```python
from build123d import *

# Parameters (mm, degrees)
SKETCH1_W            = 6
SKETCH1_H            = 6
EXTRUDE1_DEPTH       = 3.4
SKETCH2_W            = 1.5
SKETCH2_H            = 3
SKETCH2_H_2          = 0.5
SKETCH2_W_2          = 2
SKETCH2_H_3          = 6
SKETCH2_W_3          = 1
EXTRUDE2_DEPTH       = 0.4
REVOLVE1_ANGLE       = 180
LPATTERN1_COUNT      = 2
LPATTERN1_PITCH      = 4.5
LPATTERN1_COUNT_DIR2 = 2
LPATTERN1_PITCH_DIR2 = 4.5
SKETCH4_R            = 1.8
EXTRUDE3_DEPTH       = 6.1
EXTRUDE3_TAPER       = 2
EXTRUDE4_DEPTH       = 0.375
MIRROR2_COPY_1_DEPTH = 0.375
FILLET1_R            = 0.25


with BuildPart() as part:
    # Sketch1 → Extrude1 (new body)
    with BuildSketch(Plane(origin=(0, 0, 0), x_dir=(1, 0, 0), z_dir=(0, 1, 0))):
        Rectangle(SKETCH1_W, SKETCH1_H)
    extrude(amount=EXTRUDE1_DEPTH)

    # Sketch2 → Extrude2 (cut)
    with BuildSketch(Plane.XZ):
        with Locations((-2.25, 0)):
            Rectangle(SKETCH2_W, SKETCH2_H)
        with Locations((-2.25, -2.75)):
            Rectangle(SKETCH2_W, SKETCH2_H_2)
        with Locations((-2.25, 2.75)):
            Rectangle(SKETCH2_W, SKETCH2_H_2)
        Rectangle(SKETCH2_W_2, SKETCH2_H_3)
        with Locations((0, -2.25)):
            Rectangle(SKETCH2_W_3, SKETCH2_H_2, mode=Mode.SUBTRACT)
        with Locations((0, 2.25)):
            Rectangle(SKETCH2_W_3, SKETCH2_H_2, mode=Mode.SUBTRACT)
        Rectangle(SKETCH2_W_3, SKETCH2_H_2, mode=Mode.SUBTRACT)
        with Locations((2.25, 2.75)):
            Rectangle(SKETCH2_W, SKETCH2_H_2)
        with Locations((2.25, -2.75)):
            Rectangle(SKETCH2_W, SKETCH2_H_2)
        with Locations((2.25, 0)):
            Rectangle(SKETCH2_W, SKETCH2_H)
    extrude(amount=-EXTRUDE2_DEPTH, mode=Mode.SUBTRACT)

    # Sketch3 → Revolve1 (revolve)
    with BuildSketch(Plane(origin=(0, 3.4, 0), x_dir=(1, 0, 0), z_dir=(0, 1, 0))):
        with BuildLine():
            Line((-2.25, 1.75), (-2.25, 2.75))
            ThreePointArc((-2.25, 2.75), (-2.75, 2.25), (-2.25, 1.75))
        make_face()
    revolve1 = revolve(axis=Axis((-2.25, 3.4, -1.75), (0, 0, -1)), revolution_arc=REVOLVE1_ANGLE)

    # LPattern1: Revolve1 2 × 2
    with Locations(*[(i * LPATTERN1_PITCH, 0, j * LPATTERN1_PITCH_DIR2) for i in range(LPATTERN1_COUNT) for j in range(LPATTERN1_COUNT_DIR2) if (i, j) != (0, 0)]):
        add(revolve1)

    # Sketch4 → Extrude3 (add)
    with BuildSketch(Plane(origin=(0, 3.4, 0), x_dir=(1, 0, 0), z_dir=(0, 1, 0))):
        Circle(SKETCH4_R)
    extrude(amount=EXTRUDE3_DEPTH, taper=EXTRUDE3_TAPER)

    # Sketch5 → Extrude4 (add, symmetric)
    with BuildSketch(Plane(origin=(2.25, 0, 0), x_dir=(0, 0, -1), z_dir=(1, 0, 0))):
        with BuildLine():
            Line((3.125, -3.5), (3.125, -3.172113494))
            ThreePointArc((3.125, -3.172113494), (3.171283049, -2.871407695), (3.305847956, -2.598537058))
            Line((3.305847956, -2.598537058), (3.819675491, -1.864715287))
            ThreePointArc((3.819675491, -1.864715287), (3.855845082, -1.75), (3.819675491, -1.635284713))
            Line((3.819675491, -1.635284713), (3.305847956, -0.901462942))
            ThreePointArc((3.305847956, -0.901462942), (3.171283049, -0.628592305), (3.125, -0.327886506))
            Line((3.125, -0.327886506), (3.125, 0.4))
            ThreePointArc((3.125, 0.4), (3.095710678, 0.470710678), (3.025, 0.5))
            Line((3.025, 0.5), (3, 0.5))
            Line((3, 0.5), (3, 0.75))
            Line((3, 0.75), (3.025, 0.75))
            ThreePointArc((3.025, 0.75), (3.272487373, 0.647487373), (3.375, 0.4))
            Line((3.375, 0.4), (3.375, -0.327886506))
            ThreePointArc((3.375, -0.327886506), (3.409712287, -0.553415856), (3.510635967, -0.758068833))
            Line((3.510635967, -0.758068833), (4.024463502, -1.491890604))
            ThreePointArc((4.024463502, -1.491890604), (4.105845082, -1.75), (4.024463502, -2.008109396))
            Line((4.024463502, -2.008109396), (3.510635967, -2.741931167))
            ThreePointArc((3.510635967, -2.741931167), (3.409712287, -2.946584144), (3.375, -3.172113494))
            Line((3.375, -3.172113494), (3.375, -3.5))
            Line((3.375, -3.5), (3.125, -3.5))
        make_face()
    extrude4 = extrude(amount=EXTRUDE4_DEPTH, both=True)

    # Mirror1: Extrude4 across plane
    add(extrude4.mirror(Plane.XY))

    # Mirror2: Extrude4 across plane
    add(extrude4.mirror(Plane(origin=(0, 0, 0), x_dir=(0, 0, 1), z_dir=(1, 0, 0))))

    # Mirror2 copy 1 sketch → Mirror2 copy 1 (add, symmetric)
    with BuildSketch(Plane.ZY.offset(2.25)):
        with BuildLine():
            Line((3.125, -3.5), (3.125, -3.172113494))
            ThreePointArc((3.125, -3.172113494), (3.171283049, -2.871407695), (3.305847956, -2.598537058))
            Line((3.305847956, -2.598537058), (3.819675491, -1.864715287))
            ThreePointArc((3.819675491, -1.864715287), (3.855845082, -1.75), (3.819675491, -1.635284713))
            Line((3.819675491, -1.635284713), (3.305847956, -0.901462942))
            ThreePointArc((3.305847956, -0.901462942), (3.171283049, -0.628592305), (3.125, -0.327886506))
            Line((3.125, -0.327886506), (3.125, 0.4))
            ThreePointArc((3.125, 0.4), (3.095710678, 0.470710678), (3.025, 0.5))
            Line((3.025, 0.5), (3, 0.5))
            Line((3, 0.5), (3, 0.75))
            Line((3, 0.75), (3.025, 0.75))
            ThreePointArc((3.025, 0.75), (3.272487373, 0.647487373), (3.375, 0.4))
            Line((3.375, 0.4), (3.375, -0.327886506))
            ThreePointArc((3.375, -0.327886506), (3.409712287, -0.553415856), (3.510635967, -0.758068833))
            Line((3.510635967, -0.758068833), (4.024463502, -1.491890604))
            ThreePointArc((4.024463502, -1.491890604), (4.105845082, -1.75), (4.024463502, -2.008109396))
            Line((4.024463502, -2.008109396), (3.510635967, -2.741931167))
            ThreePointArc((3.510635967, -2.741931167), (3.409712287, -2.946584144), (3.375, -3.172113494))
            Line((3.375, -3.172113494), (3.375, -3.5))
            Line((3.375, -3.5), (3.125, -3.5))
        make_face()
    extrude(amount=MIRROR2_COPY_1_DEPTH, both=True)

    # Fillet1
    fillet1_edges = [part.edges().sort_by_distance(p)[0] for p in [
        (-1.586983306, 9.5, 0),
        (3, 1.9, 3),
        (-3, 1.9, 3),
        (-3, 1.9, -3),
        (3, 1.9, -3),
        (3, 1.9, 3),
        (-3, 1.9, 3),
        (-3, 1.9, -3),
        (3, 1.9, -3),
    ]]
    fillet(fillet1_edges, radius=FILLET1_R)


solid = part.part
```
Source: CAD feature listing. Evaluate the final solid. Frame: model axes, mm. A direction names the side the tool comes from. Coordinates: 2 decimals unless noted, no trailing zeros. Order: outer loops, then holes, each group sorted by start corner. A loop starts at its lowest first (then second) coordinate and runs counter-clockwise, first axis right, second up. Notation, with made-up numbers: (82, 20.25) - (140, 20.25) arc R14 cw to (140, 29.25) - close; hole circle Ø2 at (12.5, -17). An arc over 180 degrees is marked (long way). One line per item, written item: value.
1) Cut plane B-B on y = 2.5. Output: boundary loops of the cut face in (x, z).
Computed values:
outline: (-3, -2.75) arc R0.25 ccw to (-2.75, -3) - (2.75, -3) arc R0.25 ccw to (3, -2.75) - (3, 2.75) arc R0.25 ccw to (2.75, 3) - (-2.75, 3) arc R0.25 ccw to (-3, 2.75) - close
2) Reachability of faces 1 (the face through (2, 0.4, 0)), 2 (the face through (-1.3, 0, 0)), 3 (the face through (-2, 0.4, 0)), 4 (the face through (0, 9.5, 0)), 5 (the face through (-0.368, 6.37, 1.656)) from +Z, -Z, +X, -X, +Y, -Y: full face, straight path, thin tool, end or side. Return the list, or none.
Computed values:
face 1: +X, -Y
face 2: +X, -X, -Y
face 3: -X, -Y
face 4: +Z, -Z, +X, -X, +Y
face 5: +Y
3) Cut plane A-A on x = 0. Output: boundary loops of the cut face in (y, z).
Computed values:
outline: (0, -2.5) - (0.4, -2.5) - (0.4, -3) - (3.4, -3) - (3.4, -1.8) - (9.26, -1.6) arc R0.25 ccw to (9.5, -1.35) - (9.5, 1.35) arc R0.25 ccw to (9.26, 1.6) - (3.4, 1.8) - (3.4, 3) - (0.4, 3) - (0.4, 2.5) - (0, 2.5) - (0, 2) - (0.4, 2) - (0.4, 0.25) - (0, 0.25) - (0, -0.25) - (0.4, -0.25) - (0.4, -2) - (0, -2) - close
4) Mould query, pull axis X, two halves, no side actions, for faces 6 (the face through (-1.4, 3.4, -1.4)), 7 (the face through (1.3, 0, 0)), 8 (the face through (0, 0.4, -1)), 9 (the face through (-3, 2, 0)). Classes: released by +X, released by -X, zero draft, split by the parting line, or undercut.
Computed values:
face 6: undercut
face 7: zero draft
face 8: undercut
face 9: released by -X
5) Contact query for flat-ended pins moving along their axis: pin 1 (2.5 mm diameter, centred on x = -1, y = 2, fed in from -Z); pin 2 (0.8 mm diameter, centred on x = 2, y = 0, fed in from +Z); pin 3 (1.2 mm diameter, centred on y = -0.5, z = -4, fed in from +X) (3 decimals). Output: stop coordinate, or through.
Computed values:
pin 1: stops at z = -3
pin 2: stops at z = 3.38
pin 3: stops at x = 2.625
6) Ray query, line 1 (Y direction, x = -2.2, z = -0.75); line 2 (Z direction, x = 2.75, y = 3); line 3 (Y direction, x = 2.35, z = -3.5). Return the intervals inside material, ascending. Write a range as [from, to].
Computed values:
line 1: y = [0.4, 3.4]
line 2: z = [-3, 3]
line 3: y = [-2.76, -2.32], [-1.18, -0.74]
